from build123d import *

# Parameters (mm, degrees)
SKETCH1_W           = 400
SKETCH1_H           = 500
BOSS_EXTRUDE1_DEPTH = 4
SKETCH2_W           = 124
SKETCH2_H           = 235
CUT_EXTRUDE1_DEPTH  = 5
SKETCH4_R           = 2.75
CUT_EXTRUDE3_DEPTH  = 10
SKETCH5_R           = 2.5
CUT_EXTRUDE4_DEPTH  = 5
SKETCH6_R           = 2.5
CUT_EXTRUDE5_DEPTH  = 4
SKETCH7_R           = 2.75
CUT_EXTRUDE6_DEPTH  = 4
SKETCH9_W           = 124
SKETCH9_H           = 80
CUT_EXTRUDE9_DEPTH  = 4
CHAMFER1_SIZE       = 10


with BuildPart() as part:
    # Sketch1 → Boss-Extrude1 (new body)
    with BuildSketch(Plane.XY):
        with Locations((200, 250)):
            Rectangle(SKETCH1_W, SKETCH1_H)
    extrude(amount=BOSS_EXTRUDE1_DEPTH)

    # Sketch2 → Cut-Extrude1 (cut, through all)
    with BuildSketch(Plane.XY.offset(4)):
        with Locations((200, 182.5)):
            Rectangle(SKETCH2_W, SKETCH2_H)
    extrude(amount=-CUT_EXTRUDE1_DEPTH, mode=Mode.SUBTRACT)

    # Sketch4 → Cut-Extrude3 (cut)
    with BuildSketch(Plane.XY.offset(4)):
        with Locations((299, 330)):
            Circle(SKETCH4_R)
        with Locations((267, 330)):
            Circle(SKETCH4_R)
        with Locations((133, 330)):
            Circle(SKETCH4_R)
        with Locations((101, 330)):
            Circle(SKETCH4_R)
    extrude(amount=-CUT_EXTRUDE3_DEPTH, mode=Mode.SUBTRACT)

    # Sketch5 → Cut-Extrude4 (cut, through all)
    with BuildSketch(Plane.XY.offset(4)):
        with Locations((180, 319)):
            Circle(SKETCH5_R)
        with Locations((220, 319)):
            Circle(SKETCH5_R)
    extrude(amount=-CUT_EXTRUDE4_DEPTH, mode=Mode.SUBTRACT)

    # Sketch6 → Cut-Extrude5 (cut)
    with BuildSketch(Plane.XY.offset(4)):
        with Locations((72, 409.5)):
            Circle(SKETCH6_R)
        with Locations((46, 409.5)):
            Circle(SKETCH6_R)
        with Locations((72, 291.5)):
            Circle(SKETCH6_R)
        with Locations((46, 291.5)):
            Circle(SKETCH6_R)
        with Locations((328, 291.5)):
            Circle(SKETCH6_R)
        with Locations((354, 291.5)):
            Circle(SKETCH6_R)
        with Locations((328, 409.5)):
            Circle(SKETCH6_R)
        with Locations((354, 409.5)):
            Circle(SKETCH6_R)
    extrude(amount=-CUT_EXTRUDE5_DEPTH, mode=Mode.SUBTRACT)

    # Sketch7 → Cut-Extrude6 (cut)
    with BuildSketch(Plane(origin=(0, 0, 0), x_dir=(-1, 0, 0), z_dir=(0, 0, -1))):
        with Locations((-267, 20)):
            Circle(SKETCH7_R)
        with Locations((-299, 20)):
            Circle(SKETCH7_R)
        with Locations((-133, 20)):
            Circle(SKETCH7_R)
        with Locations((-101, 20)):
            Circle(SKETCH7_R)
    extrude(amount=-CUT_EXTRUDE6_DEPTH, mode=Mode.SUBTRACT)

    # Sketch9 → Cut-Extrude9 (cut)
    with BuildSketch(Plane(origin=(0, 0, 0), x_dir=(-1, 0, 0), z_dir=(0, 0, -1))):
        with Locations((-200, 400)):
            Rectangle(SKETCH9_W, SKETCH9_H)
    extrude(amount=-CUT_EXTRUDE9_DEPTH, mode=Mode.SUBTRACT)

    # Chamfer1
    chamfer1_edges = [part.edges().sort_by_distance(p)[0] for p in [
        (138, 440, 2),
        (138, 360, 2),
        (262, 360, 2),
        (262, 440, 2),
        (138, 300, 2),
        (262, 300, 2),
        (262, 65, 2),
        (138, 65, 2),
    ]]
    chamfer(chamfer1_edges, length=CHAMFER1_SIZE)


solid = part.part
Geometry check sheet. Reference: the model listing, model coordinates, mm. A direction names the side the tool comes from. Give positions to 0.01 mm unless a question says otherwise; leave off trailing zeros. Order: outer loops, then holes, each group sorted by start corner. A loop starts at its lowest first (then second) coordinate and runs counter-clockwise, first axis right, second up.
1) Material ranges on probe 1 along Y at (x, z) = (267, 3.2); probe 2 along Y at (x, z) = (220, 1.05); probe 3 along Y at (x, z) = (174.5, 2.75), recorded low to high.
Results are:
probe 1: y = 0 to 17.25, 22.75 to 327.25, 332.75 to 500
probe 2: y = 0 to 65, 300 to 316.5, 321.5 to 360, 440 to 500
probe 3: y = 0 to 65, 300 to 360, 440 to 500
2) Cross-section at A-A (y = 254). Record the boundary of the cut face in (x, z).
Results are:
outline: (0, 0) - (138, 0) - (138, 4) - (0, 4) - close; (262, 0) - (400, 0) - (400, 4) - (262, 4) - close
3) Gauge pin test, flat ends, axial feed: pin 1 (1.2 mm diameter, centred on y = 140, z = 1.5, fed in from -X); pin 2 (4.5 mm diameter, centred on x = 328, y = 291.5, fed in from +Z). Record the tip position at first contact, or that the pin passes through.
Results are:
pin 1: stops at x = 0
pin 2: passes through
4) Tool access check on faces 3 (the flat face through (143, 435, 2)), 4 (the flat face through (197, 309, 0)). Record the directions out of +Z, -Z, +X, -X, +Y, -Y that give a thin tool (end or side, any length) a straight path to the whole face; none if there is none.
Results are:
face 3: +Z, -Z
face 4: -Z, +X, -X, +Y, -Y
5) Draft check along Y on faces 1 (the flat face through (197, 309, 4)), 2 (the flat face through (143, 70, 2)). Enter one of: released by +Y, released by -Y, zero draft, split by the parting line, or undercut.
Results are:
face 1: zero draft
face 2: undercut
6) Cross-section at B-B (z = 1.5). Give the number of separate pieces and of enclosed holes in the cut face, then the cut area to 3 significant figures.
Results are:
separate pieces: 1
enclosed holes: 20
area: 161,000 mm2
